Autodesk Fusion 360 part; units mm, degrees
sketch "Schizzo1" plane through (0, 0, 0) normal (0, 0, 1) x (1, 0, 0)
  line L0 (30, -30) -> (-30, -30)
  line L1 (-30, -30) -> (-30, 30)
  line L2 (-30, 30) -> (30, 30)
  line L3 (30, 30) -> (30, -30)
  line L4 (30, -30) -> (-30, 30) construction
  line L5 (-30, -30) -> (30, 30) construction
  line L6 (22.5, -28) -> (-22.5, -28)
  line L7 (-28, -22.5) -> (-28, 22.5)
  line L8 (-22.5, 28) -> (22.5, 28)
  line L9 (28, 22.5) -> (28, -22.5)
  arc A0 (-22.5, 28) -> (-28, 22.5) centre (-22.5, 22.5) ccw
  arc A1 (28, 22.5) -> (22.5, 28) centre (22.5, 22.5) ccw
  arc A2 (22.5, -28) -> (28, -22.5) centre (22.5, -22.5) ccw
  arc A3 (-28, -22.5) -> (-22.5, -28) centre (-22.5, -22.5) ccw
  dimension "d1" = 60
  dimension "d2" = 60
  dimension "d4" = 5.5
extrude "Estrusione1" add sketch "Schizzo1" along normal blind 30 contours L6 L7 L8 L9 A0 A1 A2 A3
sketch "Schizzo2" plane through (0, 0, 30) normal (0, 0, 1) x (-1, 0, 0)
  arc A0 (22.5, -28) -> (28, -22.5) centre (22.5, -22.5) ccw
  line L0 (28, -22.5) -> (28, 22.5)
  arc A1 (28, 22.5) -> (22.5, 28) centre (22.5, 22.5) ccw
  line L1 (22.5, 28) -> (-22.5, 28)
  arc A2 (-22.5, 28) -> (-28, 22.5) centre (-22.5, 22.5) ccw
  line L2 (-28, 22.5) -> (-28, -22.5)
  arc A3 (-28, -22.5) -> (-22.5, -28) centre (-22.5, -22.5) ccw
  line L3 (-22.5, -28) -> (22.5, -28)
  line L4 (15, -28) -> (15, -23)
  line L5 (20, -18) -> (28, -18)
  arc A4 (20, -18) -> (15, -23) centre (20, -23) ccw
  dimension "d7" = 5
  dimension "d8" = 13
  dimension "d9" = 10
extrude "Estrusione2" cut sketch "Schizzo2" against normal blind 8 contours A0 L0 L3 L4 L5 A4
pattern_circular "Serie C1" count 2 over 360 about axis through (0, 0, 1.75) along (0, 0, 1) of "Estrusione2"
sketch "Schizzo3" plane through (0, 0, 30) normal (0, 0, 1) x (-1, 0, 0)
  line L0 (-20, 18) -> (-28, 18)
  line L1 (-28, 18) -> (-28, -22.5)
  arc A0 (-28, -22.5) -> (-22.5, -28) centre (-22.5, -22.5) ccw
  line L2 (-22.5, -28) -> (15, -28)
  line L3 (15, -28) -> (15, -23)
  arc A1 (20, -18) -> (15, -23) centre (20, -23) ccw
  line L4 (20, -18) -> (28, -18)
  line L5 (28, -18) -> (28, 22.5)
  arc A2 (28, 22.5) -> (22.5, 28) centre (22.5, 22.5) ccw
  line L6 (22.5, 28) -> (-15, 28)
  line L7 (-15, 28) -> (-15, 23)
  arc A3 (-20, 18) -> (-15, 23) centre (-20, 23) ccw
  line L8 (10, -28) -> (10, -7)
  line L9 (14, -3) -> (28, -3)
  line L10 (-2, -28) -> (-2, 5)
  line L11 (2, 9) -> (28, 9)
  arc A4 (14, -3) -> (10, -7) centre (14, -7) ccw
  arc A5 (2, 9) -> (-2, 5) centre (2, 5) ccw
  circle A6 centre (-13, -15) radius 7.5
  circle A7 centre (23, -23) radius 3
  circle A8 centre (-23, 23) radius 3
  line L12 (28, 15) -> (-2, 15)
  line L13 (-7, 20) -> (-7, 28)
  arc A9 (-7, 20) -> (-2, 15) centre (-2, 20) ccw
  point P0 (-28, 18)
  dimension "d14" = 12
  dimension "d15" = 18
  dimension "d16" = 25
  dimension "d17" = 12
  dimension "d18" = 4
  dimension "d19" = 15
  dimension "d20" = 6
  dimension "d21" = 6
  dimension "d22" = 5
  dimension "d23" = 5
  dimension "d24" = 5
  dimension "d25" = 5
  dimension "d26" = 13
  dimension "d27" = 15
  dimension "d28" = 13
  dimension "d29" = 35
  dimension "d30" = 5
extrude "Estrusione3" cut sketch "Schizzo3" against normal blind 85 contours A7 | A8
extrude "Estrusione4" cut sketch "Schizzo3" against normal blind 15 contours A6
extrude "Estrusione5" cut sketch "Schizzo3" against normal blind 8 contours L2 L5 L8 L9 L10 L11 A4 A5
extrude "Estrusione6" cut sketch "Schizzo3" against normal blind 10 contours L5 A2 L6 L12 L13 A9
delete_face "EliminaFaccia1" 1 faces at (-27.845, -23.7967, 13.3333)
delete_face "EliminaFaccia2" 1 faces at (26.4805, 26.2954, 20)
chamfer "Smusso1" distance 3.5 angle 45 1 edges at (28, 28, 15)
chamfer "Smusso2" distance 8 angle 45 1 edges at (-28, -28, 10)
chamfer "Smusso3" distance 1 angle 45 10 edges at (-28, -15, 25) (-28, -9, 26) (-28, 3, 26) (-28, 18, 26) (-15, 28, 26) (-10, 28, 26) (2, 28, 26) (15, -28, 26) (28, -18, 26) (7, -28, 25)
chamfer "Smusso6" distance 1 angle 45 1 edges at (19.9925, 12.2879, 30)
Input: part model. Units: mm. Frame: model coordinates. A direction names the side the tool comes from. Give positions to 0.01 mm unless a question says otherwise; leave off trailing zeros. Order: outer loops, then holes, each group sorted by start corner. A loop starts at its lowest first (then second) coordinate and runs counter-clockwise, first axis right, second up. Notation, with made-up numbers: (51.5, 17) - (55.5, 17) arc R21 cw to (55.5, 55) - close; hole circle Ø4 at (-32.75, 58.5). An arc over 180 degrees is marked (long way). Answer as a JSON object with one key per item and string values. Group by question number.
Q1. First-contact query: pin 1 Ø11 at (x, z) = (-17.5, 27.5) entering from -Y; pin 2 Ø3.5 at (x, z) = (-22, 27.5) entering from +Y; pin 3 Ø4.5 at (y, z) = (-25, 24.5) entering from +X. Flat tips, straight axial feed; report the tip coordinate or a pass-through.
Q2. Mould query, pull axis Y, two halves, no side actions, for faces 4 (the face through (19, -22, 22)), 5 (the face through (1, 28, 15)), 6 (the face through (-14, -9, 26)), 7 (the face through (-24, -24, 10)). Classes: pulls with the +Y half, pulls with the -Y half, needs draft (parallel to the pull), parting line crosses it, or undercut.
Q3. Cut plane C-C, the plane y = 15. Output: boundary loops of the cut face in (x, z), then the cut area to 3 significant figures.
Q4. Cut plane A-A, the plane z = 23.5. Count the separate pieces of the cut face and the enclosed holes in it, then the cut area to 3 significant figures.
Q5. Cut plane D-D, the plane x = -23.5. Output: boundary loops of the cut face in (y, z).
Q6. Cut plane B-B, the plane x = -9. Output: boundary loops of the cut face in (y, z).
Q7. Line query: probe 1 along X at (y, z) = (15, 25); probe 2 along Y at (x, z) = (-23, 25.5); probe 3 along X at (y, z) = (23, 15.75). Output: solid intervals per line, ascending.
Q8. Set-up query: faces 1 (the face through (-19, 22, 22)), 2 (the face through (-11.203, 4.141, 26.056)), 3 (the face through (17, -19, 26)). Return all of +Z, -Z, +X, -X, +Y, -Y with unobstructed straight access to the full face (end or side cutting, diameter ignored); none if empty.
Results:
{
 "1": {"pin 1": "y = -15", "pin 2": "y = 18", "pin 3": "x = 15.01"},
 "2": {"face 4": "needs draft", "face 5": "pulls with the +Y half", "face 6": "undercut", "face 7": "pulls with the -Y half"},
 "3": {"outline": "(-28, 0) - (28, 0) - (28, 30) - (21.5, 30) - (20.5, 29) - (20.5, 15) - (5.5, 15) - (5.5, 29) - (4.5, 30) - (2, 30) - (2, 22) - (-10, 22) - (-10, 30) - (-28, 30) - close", "area": "1,360 mm^2"},
 "4": {"separate pieces": "2", "enclosed holes": "1", "area": "1,590 mm^2"},
 "5": {"outline": "(-24.5, 0) - (20.04, 0) - (20.04, 22) - (18, 22) - (18, 30) - (3, 30) - (3, 22) - (-9, 22) - (-9, 30) - (-15, 30) - (-15, 20) - (-24.5, 20) - close; (25.96, 0) - (27.91, 0) - (27.91, 22) - (25.96, 22) - close"},
 "6": {"outline": "(-28, 0) - (28, 0) - (28, 22) - (-9, 22) - (-9, 30) - (-15, 30) - (-15, 20) - (-28, 20) - close"},
 "7": {"probe 1": "-28 to -10, 2 to 5.5, 20.5 to 28", "probe 2": "-15 to -9, 3 to 18", "probe 3": "-27.98 to -26, -20 to 28"},
 "8": {"face 1": "+Z, -X, +Y", "face 2": "+Z", "face 3": "+Z, +X, -Y"}
}
